from build123d import *

# Parameters (mm, degrees)
SKETCH_1_R      = 1.6
SKETCH_1_W      = 10.1
SKETCH_1_H      = 10
EXTRUDE_1_DEPTH = 10


with BuildPart() as part:
    # Эскиз1 → Бобышка-Вытянуть1 (new body)
    with BuildSketch(Plane.XY):
        with BuildLine():
            Line((-37.4993057, -208.951162), (-37.4993057, 208.951162))
            Line((-37.4993057, 208.951162), (27.5006943, 208.951162))
            Line((27.5006943, 208.951162), (27.5006943, 155.851162))
            Line((27.5006943, 155.851162), (37.4993057, 155.684518477))
            Line((37.4993057, 155.684518477), (37.4993057, 145.684518477))
            Line((37.4993057, 145.684518477), (27.5006943, 145.651162))
            Line((27.5006943, 145.651162), (27.5006943, 117.301162))
            Line((27.5006943, 117.301162), (20.7006943, 117.301162))
            Line((20.7006943, 117.301162), (20.7006943, 118.501162))
            Line((20.7006943, 118.501162), (18.5006943, 118.501162))
            Line((18.5006943, 118.501162), (18.5006943, 117.301162))
            Line((18.5006943, 117.301162), (17.0006943, 117.301162))
            Line((17.0006943, 117.301162), (17.0006943, 114.201162))
            Line((17.0006943, 114.201162), (18.5006943, 114.201162))
            Line((18.5006943, 114.201162), (18.5006943, 113.001162))
            Line((18.5006943, 113.001162), (20.7006943, 113.001162))
            Line((20.7006943, 113.001162), (20.7006943, 114.201162))
            Line((20.7006943, 114.201162), (27.5006943, 114.201162))
            Line((27.5006943, 114.201162), (27.5006943, 85.851162))
            Line((27.5006943, 85.851162), (37.4993057, 85.684518477))
            Line((37.4993057, 85.684518477), (37.4993057, 75.684518477))
            Line((37.4993057, 75.684518477), (27.5006943, 75.651162))
            Line((27.5006943, 75.651162), (27.5006943, -94.148838))
            Line((27.5006943, -94.148838), (37.4993057, -94.315481523))
            Line((37.4993057, -94.315481523), (37.4993057, -104.315481523))
            Line((37.4993057, -104.315481523), (27.5006943, -104.348838))
            Line((27.5006943, -104.348838), (27.5006943, -132.698838))
            Line((27.5006943, -132.698838), (20.7006943, -132.698838))
            Line((20.7006943, -132.698838), (20.7006943, -131.498838))
            Line((20.7006943, -131.498838), (18.5006943, -131.498838))
            Line((18.5006943, -131.498838), (18.5006943, -132.698838))
            Line((18.5006943, -132.698838), (17.0006943, -132.698838))
            Line((17.0006943, -132.698838), (17.0006943, -135.798838))
            Line((17.0006943, -135.798838), (18.5006943, -135.798838))
            Line((18.5006943, -135.798838), (18.5006943, -136.998838))
            Line((18.5006943, -136.998838), (20.7006943, -136.998838))
            Line((20.7006943, -136.998838), (20.7006943, -135.798838))
            Line((20.7006943, -135.798838), (27.5006943, -135.798838))
            Line((27.5006943, -135.798838), (27.5006943, -164.148838))
            Line((27.5006943, -164.148838), (37.4993057, -164.315481523))
            Line((37.4993057, -164.315481523), (37.4993057, -174.315481523))
            Line((37.4993057, -174.315481523), (27.5006943, -174.348838))
            Line((27.5006943, -174.348838), (27.5006943, -208.951162))
            Line((27.5006943, -208.951162), (0.6006943, -208.951162))
            Line((0.6006943, -208.951162), (0.6006943, -202.951162))
            ThreePointArc((0.6006943, -202.951162), (0.014907862, -201.536948438), (-1.3993057, -200.951162))
            Line((-1.3993057, -200.951162), (-5.3993057, -200.951162))
            ThreePointArc((-5.3993057, -200.951162), (-6.813519263, -201.536948438), (-7.3993057, -202.951162))
            Line((-7.3993057, -202.951162), (-7.3993057, -208.951162))
            Line((-7.3993057, -208.951162), (-19.3993057, -208.951162))
            Line((-19.3993057, -208.951162), (-19.3993057, -202.151162))
            Line((-19.3993057, -202.151162), (-18.1993057, -202.151162))
            Line((-18.1993057, -202.151162), (-18.1993057, -199.951162))
            Line((-18.1993057, -199.951162), (-19.3993057, -199.951162))
            Line((-19.3993057, -199.951162), (-19.3993057, -198.451162))
            Line((-19.3993057, -198.451162), (-22.4993057, -198.451162))
            Line((-22.4993057, -198.451162), (-22.4993057, -199.951162))
            Line((-22.4993057, -199.951162), (-23.6993057, -199.951162))
            Line((-23.6993057, -199.951162), (-23.6993057, -202.151162))
            Line((-23.6993057, -202.151162), (-22.4993057, -202.151162))
            Line((-22.4993057, -202.151162), (-22.4993057, -208.951162))
            Line((-22.4993057, -208.951162), (-37.4993057, -208.951162))
        make_face()
        with Locations((-29.9493057, 115.851162)):
            Circle(SKETCH_1_R, mode=Mode.SUBTRACT)
        with Locations((-29.9493057, -134.148838)):
            Circle(SKETCH_1_R, mode=Mode.SUBTRACT)
        with Locations((-29.9493057, 150.851162)):
            Rectangle(SKETCH_1_W, SKETCH_1_H, mode=Mode.SUBTRACT)
        with Locations((-29.9493057, -169.148838)):
            Rectangle(SKETCH_1_W, SKETCH_1_H, mode=Mode.SUBTRACT)
        with Locations((-29.9493057, 80.851162)):
            Rectangle(SKETCH_1_W, SKETCH_1_H, mode=Mode.SUBTRACT)
        with Locations((-29.9493057, -99.148838)):
            Rectangle(SKETCH_1_W, SKETCH_1_H, mode=Mode.SUBTRACT)
    extrude(amount=EXTRUDE_1_DEPTH)


solid = part.part
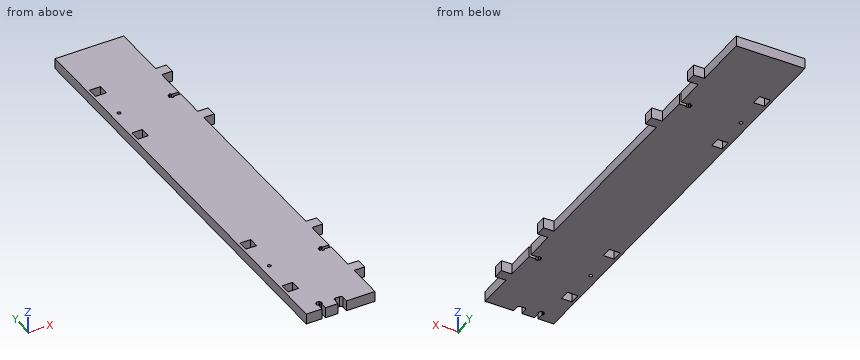
Build history of the part. All positions in model axes, mm. Coordinates: 2 decimals unless noted, no trailing zeros. Order: outer loops, then holes, each group sorted by start corner. A loop starts at its lowest first (then second) coordinate and runs counter-clockwise, first axis right, second up. Notation, with made-up numbers: M 51.25,25.5 L 62.25,25.5 A7 ccw 62.25,35.5 Z; hole C 31,47.25 d1. An arc over 180 degrees is marked long. One line per question, with ' | ' between items. Start each with the question number.
Q1. Saw through at B-B (z = 3). Count the separate pieces of the cut face and the enclosed holes in it, then the cut area to 3 significant figures.
Q2. Flat gauge pins, fed straight in: pin 1 Ø0.6 at (y, z) = (-132.5, 3) entering from +X; pin 2 Ø5 at (x, y) = (-24, -73) entering from -Z; pin 3 Ø2.5 at (x, y) = (-29.95, 115.85) entering from -Z. Where does each tip first touch, or does it go through?
Q3. Saw through at A-A (y = -0.5). List the corners of the cut face in (x, z).
Q4. Probe L1, parallel to Y at x = -26, z = 7.5; L2, parallel to Y at x = 20.5, z = 1.5; L3, parallel to X at y = -64.5, z = 5.75. List the from-to ranges inside material, lowest first. Write a range as from..to.
Check values:
1) separate pieces: 1 | enclosed holes: 6 | area: 27,000 mm2
2) pin 1: stops at x = 27.5 | pin 2: stops at z = 0 | pin 3: passes through
3) outline: M -37.5,0 L 27.5,0 L 27.5,10 L -37.5,10 Z
4) L1: y = -208.95..-174.15, -164.15..-104.15, -94.15..75.85, 85.85..145.85, 155.85..208.95 | L2: y = -208.95..-137, -131.5..113, 118.5..208.95 | L3: x = -37.5..27.5
